Can you work these out from the model? Positions are in its coordinate system, mm. Round coordinates to 2 decimals unless told otherwise and drop trailing zeros. Write each loop counter-clockwise with the first axis right and the second up, starting at its lowest first coordinate (ties: lowest second). Pieces come first, ordered by that corner, then holes. Notation, with made-up numbers: M 85,85.5 L 138,85.5 A12 cw 138,107.5 Z; hole C 45.25,-15.75 d10. An arc over 180 degrees is marked long. Answer in a Markdown table with one row per item. Add a question column.
(1) If I drill on probe 1 along Y at (x, z) = (4.25, 4.75), over which ranges is the centre line in solid material (lowest first)?
(2) Suppose I cut it at A-A, the plane z = 5. Write out the boundary of the cut face in (x, y), then the cut area to 3 significant figures.
(3) I'm going to push a flat-ended pin straight in: pin 1 (3 mm diameter, centred on x = -3.5, y = 170.5, fed in from -Z). Where does the tip first touch, or does it pass through?
(4) Suppose I cut it at B-B, the plane x = 0. Write out the boundary of the cut face in (y, z), then the cut area to 3 significant figures.
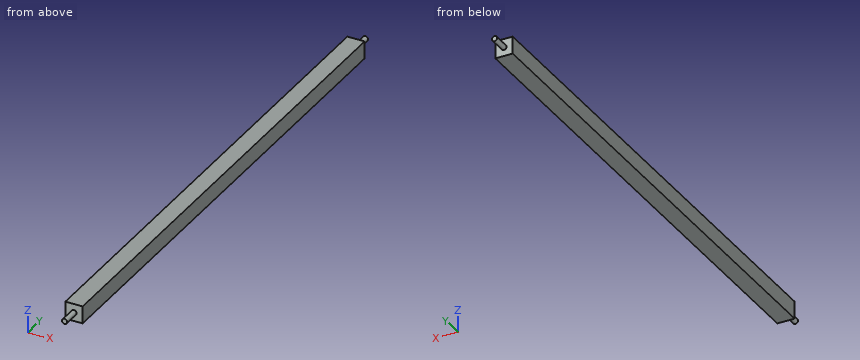
from build123d import *

# Parameters (mm, degrees)
F0_W       = 300
F0_H       = 10
F1_DEPTH   = 5
F2_R       = 1.5
F1_FACE1_W = 10
F1_FACE1_H = 10
F3_DEPTH   = 10
F4_R       = 1.5
F5_DEPTH   = 10


with BuildPart() as f1:
    # F0 (on Right) → F1 (new body, symmetric)
    with BuildSketch(Plane.YZ):
        with Locations((150, 5)):
            Rectangle(F0_W, F0_H)
    extrude(amount=F1_DEPTH, both=True)

    # F2 (on face) + F1_face1 (on face) → F3 (join)
    with BuildSketch(Plane.XZ):
        with Locations((0, 5)):
            Circle(F2_R)
    with BuildSketch(Plane(origin=(0, 300, 5), x_dir=(-1, 0, 0), z_dir=(0, 1, 0))):
        Rectangle(F1_FACE1_W, F1_FACE1_H)
    extrude(amount=F3_DEPTH, dir=(0, -1, 0))

    # F4 (on face) → F5 (join)
    with BuildSketch(Plane(origin=(0, 300, 0), x_dir=(-1, 0, 0), z_dir=(0, 1, 0))):
        with Locations((0, 5)):
            Circle(F4_R)
    extrude(amount=F5_DEPTH)


solid = f1.part
Calculated:
| question | item | result |
|---|---|---|
| 1 | probe 1 | 0 to 300 |
| 2 | outline | M -5,0 L -1.5,0 L -1.5,-10 L 1.5,-10 L 1.5,0 L 5,0 L 5,300 L 1.5,300 L 1.5,310 L -1.5,310 L -1.5,300 L -5,300 Z |
| 2 | area | 3,060 mm² |
| 3 | pin 1 | z = 0 |
| 4 | outline | M -10,3.5 L 0,3.5 L 0,0 L 300,0 L 300,3.5 L 310,3.5 L 310,6.5 L 300,6.5 L 300,10 L 0,10 L 0,6.5 L -10,6.5 Z |
| 4 | area | 3,060 mm² |
